from build123d import *

# Parameters (mm, degrees)
SKETCH1_R            = 14
SKETCH1_R_2          = 7
BOSS_EXTRUDE1_DEPTH  = 8
SKETCH1_3_R          = 23
SKETCH1_3_R_2        = 19
SKETCH1_3_R_3        = 14
BOSS_EXTRUDE2_DEPTH  = 8
SKETCH1_4_R          = 19
SKETCH1_4_R_2        = 14
BOSS_EXTRUDE3_DEPTH  = 8
SKETCH1_5_R          = 40
SKETCH1_5_R_2        = 23
BOSS_EXTRUDE4_DEPTH  = 2
BOSS_EXTRUDE5_START  = -4
SKETCH1_6_R          = 40
SKETCH1_6_R_2        = 23
BOSS_EXTRUDE5_DEPTH  = 4
BOSS_EXTRUDE6_START  = -8
SKETCH1_8_R          = 45
SKETCH1_8_R_2        = 40
BOSS_EXTRUDE6_DEPTH  = 8
SKETCH1_9_R          = 45
SKETCH1_9_R_2        = 40
BOSS_EXTRUDE7_DEPTH  = 4
BOSS_EXTRUDE8_START  = -2
SKETCH1_10_R         = 5
SKETCH1_10_R_2       = 45
BOSS_EXTRUDE8_DEPTH  = 2
SKETCH1_12_R         = 5
SKETCH1_12_R_2       = 45
BOSS_EXTRUDE10_DEPTH = 4
FILLET1_R            = 4
CHAMFER1_SIZE        = 1
FILLET2_R            = 2


with BuildPart() as part:
    # Sketch1 → Boss-Extrude1 (new body)
    with BuildSketch(Plane.XY):
        Circle(SKETCH1_R)
        Circle(SKETCH1_R_2, mode=Mode.SUBTRACT)
    extrude(amount=BOSS_EXTRUDE1_DEPTH)

    # Sketch1_3 → Boss-Extrude2 (add)
    # profile 1 of 2: a face of its own
    with BuildSketch(Plane.XY):
        Circle(SKETCH1_3_R)
        Circle(SKETCH1_3_R_2, mode=Mode.SUBTRACT)
    # profile 2 of 2: a face of its own
    with BuildSketch(Plane.XY):
        Circle(SKETCH1_3_R_2)
        Circle(SKETCH1_3_R_3, mode=Mode.SUBTRACT)
    extrude(amount=BOSS_EXTRUDE2_DEPTH)

    # Sketch1_4 → Boss-Extrude3 (add)
    with BuildSketch(Plane.XY):
        Circle(SKETCH1_4_R)
        Circle(SKETCH1_4_R_2, mode=Mode.SUBTRACT)
    extrude(amount=-BOSS_EXTRUDE3_DEPTH)

    # Sketch1_5 → Boss-Extrude4 (add)
    with BuildSketch(Plane.XY):
        Circle(SKETCH1_5_R)
        Circle(SKETCH1_5_R_2, mode=Mode.SUBTRACT)
    extrude(amount=BOSS_EXTRUDE4_DEPTH)

    # Sketch1_6 → Boss-Extrude5 (add)
    with BuildSketch(Plane.XY.offset(BOSS_EXTRUDE5_START)):
        Circle(SKETCH1_6_R)
        Circle(SKETCH1_6_R_2, mode=Mode.SUBTRACT)
    extrude(amount=BOSS_EXTRUDE5_DEPTH)

    # Sketch1_8 → Boss-Extrude6 (add)
    with BuildSketch(Plane.XY.offset(BOSS_EXTRUDE6_START)):
        Circle(SKETCH1_8_R)
        Circle(SKETCH1_8_R_2, mode=Mode.SUBTRACT)
    extrude(amount=BOSS_EXTRUDE6_DEPTH)

    # Sketch1_9 → Boss-Extrude7 (add)
    with BuildSketch(Plane.XY):
        Circle(SKETCH1_9_R)
        Circle(SKETCH1_9_R_2, mode=Mode.SUBTRACT)
    extrude(amount=BOSS_EXTRUDE7_DEPTH)

    # Sketch1_10 → Boss-Extrude8 (add)
    with BuildSketch(Plane.XY.offset(BOSS_EXTRUDE8_START)):
        Polygon((-53, -30.599564267), (0, -61.199128534), (53, -30.599564267), (53, 30.599564267), (0, 61.199128534), (-53, 30.599564267), align=None)
        with Locations((-44.167295593, 25.5)):
            Circle(SKETCH1_10_R, mode=Mode.SUBTRACT)
        with Locations((-44.167295593, -25.5)):
            Circle(SKETCH1_10_R, mode=Mode.SUBTRACT)
        with Locations((0, -51)):
            Circle(SKETCH1_10_R, mode=Mode.SUBTRACT)
        with Locations((44.167295593, -25.5)):
            Circle(SKETCH1_10_R, mode=Mode.SUBTRACT)
        with Locations((44.167295593, 25.5)):
            Circle(SKETCH1_10_R, mode=Mode.SUBTRACT)
        Circle(SKETCH1_10_R_2, mode=Mode.SUBTRACT)
        with Locations((0, 51)):
            Circle(SKETCH1_10_R, mode=Mode.SUBTRACT)
    extrude(amount=BOSS_EXTRUDE8_DEPTH)

    # Sketch1_12 → Boss-Extrude10 (add)
    with BuildSketch(Plane.XY):
        Polygon((-53, -30.599564267), (0, -61.199128534), (53, -30.599564267), (53, 30.599564267), (0, 61.199128534), (-53, 30.599564267), align=None)
        with Locations((-44.167295593, 25.5)):
            Circle(SKETCH1_12_R, mode=Mode.SUBTRACT)
        with Locations((-44.167295593, -25.5)):
            Circle(SKETCH1_12_R, mode=Mode.SUBTRACT)
        with Locations((0, -51)):
            Circle(SKETCH1_12_R, mode=Mode.SUBTRACT)
        with Locations((44.167295593, -25.5)):
            Circle(SKETCH1_12_R, mode=Mode.SUBTRACT)
        with Locations((44.167295593, 25.5)):
            Circle(SKETCH1_12_R, mode=Mode.SUBTRACT)
        Circle(SKETCH1_12_R_2, mode=Mode.SUBTRACT)
        with Locations((0, 51)):
            Circle(SKETCH1_12_R, mode=Mode.SUBTRACT)
    extrude(amount=BOSS_EXTRUDE10_DEPTH)

    # Fillet1
    fillet1_edges = [part.edges().sort_by_distance(p)[0] for p in [
        (-23, 0, 2),
    ]]
    fillet(fillet1_edges, radius=FILLET1_R)

    # Chamfer1
    chamfer1_edges = [part.edges().sort_by_distance(p)[0] for p in [
        (-45, 0, -8),
    ]]
    chamfer(chamfer1_edges, length=CHAMFER1_SIZE)

    # Fillet2
    fillet2_edges = [part.edges().sort_by_distance(p)[0] for p in [
        (-26.5, -45.899346401, 4),
        (-26.5, 45.899346401, 4),
        (-53, 0, 4),
    ]]
    fillet(fillet2_edges, radius=FILLET2_R)


solid = part.part
The model under review builds one solid part; all positions refer to its coordinate system, in mm. A direction names the side the tool comes from. Round coordinates to 2 decimals unless told otherwise and drop trailing zeros. Order: outer loops, then holes, each group sorted by start corner. A loop starts at its lowest first (then second) coordinate and runs counter-clockwise, first axis right, second up. Notation, with made-up numbers: (42.5, 80) -> (82.5, 80) arc R21 ccw to (82.5, 95) -> close; hole circle Ø11 at (16, 59.5). An arc over 180 degrees is marked (long way). Use CSV: the item, a comma, the result in double quotes. Start each with the question number.
(1) Tool access review of faces 4 (the face through (-26.093, 45.476, 3.399)), 5 (the face through (-8.67, -39.05, 2.99)), 6 (the face through (3, 19, 0)): name each direction out of +Z, -Z, +X, -X, +Y, -Y from which nothing blocks a thin tool from reaching the whole face with its end or side.
(2) Consider section B-B on x = -2. State how many separate pieces and enclosed holes the cut face has, and give its area (3 significant figures).
(3) Wall thickness on probe 1 along Y at (x, z) = (0, -0.45); probe 2 along Y at (x, z) = (0, -6); probe 3 along Y at (x, z) = (-5.5, -3): over which ranges is each line inside the solid? List them lowest first. Write a range as from..to.
(4) Insertion check: pin 1 (1 mm diameter, centred on x = -5, z = 0, fed in from -Y); pin 2 (22.5 mm diameter, centred on x = 0, y = 0, fed in from -Z); pin 3 (23 mm diameter, centred on x = 5.5, y = -11.5, fed in from -Z); pin 4 (9 mm diameter, centred on x = 44.17, y = 25.5, fed in from +Z). Each pin has a flat end and moves straight along its axis. Give the tip position at first contact, or say it passes through.
(5) Mouldability with a two-part tool opening along X and no side actions: class faces 1 (the face through (-2.994, 22.804, 6.986)), 2 (the face through (-2.994, 22.804, -2.028)), 3 (the face through (-53, 0, 0)) as pulls with the +X half, pulls with the -X half, needs draft (parallel to the pull), parting line crosses it, or undercut.
(6) Consider section A-A on z = -5.5. Write out the cut boundary in (x, y), and give its area (3 significant figures).
Responses:
1,face 4,"+Z, -X, +Y"
1,face 5,"+Z"
1,face 6,"-Z"
2,separate pieces,"4"
2,enclosed holes,"0"
2,area,"739 mm²"
3,probe 1,"-61.2..-56, -46..-23, -19..-14, 14..19, 23..46, 56..61.2"
3,probe 2,"-45..-40, -19..-14, 14..19, 40..45"
3,probe 3,"-44.66..-22.33, -18.19..-12.87, 12.87..18.19, 22.33..44.66"
4,pin 1,"y = -58.6"
4,pin 2,"z = 0"
4,pin 3,"z = -8"
4,pin 4,"through"
5,face 1,"parting line crosses it"
5,face 2,"undercut"
5,face 3,"pulls with the -X half"
6,outline,"circle Ø90 at (0, 0); circle Ø38 at (0, 0); hole circle Ø80 at (0, 0); hole circle Ø28 at (0, 0)"
6,area,"1,850 mm²"
